```python
from build123d import *

# Parameters (mm, degrees)
BOSS_EXTRUDE2_DEPTH   = 3.81
BOSS_EXTRUDE2_2_DEPTH = 3.81
BOSS_EXTRUDE3_START   = 0.508
SKETCH2_3_R           = 2.794
BOSS_EXTRUDE3_DEPTH   = 2.286
BOSS_EXTRUDE11_DEPTH  = 3.81
BOSS_EXTRUDE12_DEPTH  = 0.889
BOSS_EXTRUDE14_START  = 10.16
BOSS_EXTRUDE14_DEPTH  = 50.8
BOSS_EXTRUDE17_START  = 60.071
BOSS_EXTRUDE17_DEPTH  = 0.889
SKETCH14_W            = 15.24
SKETCH14_H            = 59.182
CUT_EXTRUDE3_DEPTH    = 88.666803866


with BuildPart() as part:
    # Sketch2 → Boss-Extrude2 (new body)
    with BuildSketch(Plane(origin=(0, 0, 0), x_dir=(1, 0, 0), z_dir=(0, 1, 0))):
        Polygon((0, 7.62), (0, 0), (36.83, 0), (36.83, 7.62), (7.62, 7.62), (6.87, 7.62), align=None)
    extrude(amount=BOSS_EXTRUDE2_DEPTH)



with BuildPart() as body_2:
    # Sketch2 → Boss-Extrude2 2 (new body)
    with BuildSketch(Plane(origin=(0, 0, 0), x_dir=(1, 0, 0), z_dir=(0, 1, 0))):
        Polygon((0, 76.2), (0, 68.58), (6.87, 68.58), (7.62, 68.58), (36.83, 68.58), (36.83, 76.2), align=None)
    extrude(amount=BOSS_EXTRUDE2_2_DEPTH)


with BuildPart() as part_1:
    add(part.part)

    add(body_2.part)  # Boss-Extrude3 merges body 2
    # Sketch2<3> → Boss-Extrude3 (add)
    # profile 1 of 2: a face of its own
    with BuildSketch(Plane(origin=(0, 0, 0), x_dir=(1, 0, 0), z_dir=(0, 1, 0)).offset(BOSS_EXTRUDE3_START)):
        Polygon((0, 68.58), (0, 7.62), (6.87, 7.62), (7.62, 7.62), (36.83, 7.62), (36.83, 68.58), (7.62, 68.58), (6.87, 68.58), align=None)
        with Locations(Location((29.21, 22.86, 0), (0, 0, 270))):
            Circle(SKETCH2_3_R, mode=Mode.SUBTRACT)
        with Locations(Location((29.21, 53.34, 0), (0, 0, 270))):
            Circle(SKETCH2_3_R, mode=Mode.SUBTRACT)
    # profile 2 of 2: a face of its own
    with BuildSketch(Plane(origin=(0, 0, 0), x_dir=(1, 0, 0), z_dir=(0, 1, 0)).offset(BOSS_EXTRUDE3_START)):
        Polygon((0, 68.58), (0, 7.62), (6.87, 7.62), (7.62, 7.62), (36.83, 7.62), (36.83, 68.58), (7.62, 68.58), (6.87, 68.58), align=None)
        with Locations(Location((29.21, 22.86, 0), (0, 0, 270))):
            Circle(SKETCH2_3_R, mode=Mode.SUBTRACT)
        with Locations(Location((29.21, 53.34, 0), (0, 0, 270))):
            Circle(SKETCH2_3_R, mode=Mode.SUBTRACT)
    extrude(amount=BOSS_EXTRUDE3_DEPTH)

    # Sketch13 → Boss-Extrude11 (add)
    with BuildSketch(Plane.XY.offset(-68.58)):
        Polygon((6.215980089, 2.794), (7.231980089, 2.794), (7.231980089, 3.298518966), align=None)
        Polygon((8.120980089, 2.794), (8.120980089, 3.81), (7.231980089, 3.81), (7.231980089, 3.298518966), (7.231980089, 2.794), align=None)
        Polygon((8.120980089, 3.81), (8.120980089, 22.975432281), (8.120980089, 24.638), (9.046534916, 24.638), (19.649280137, 24.638), (20.820980089, 24.638), (21.060045846, 22.582034491), (23.242840554, 3.81), (24.261745737, 3.81), (21.784207173, 25.654), (7.231980089, 25.654), (7.231980089, 3.81), align=None)
        Polygon((8.120980089, 24.638), (8.120980089, 22.975432281), (9.046534916, 24.638), align=None)
        Polygon((20.820980089, 24.638), (19.649280137, 24.638), (21.060045846, 22.582034491), align=None)
        Polygon((24.261745737, 3.81), (23.242840554, 3.81), (23.360980089, 2.794), (24.376980089, 2.794), (24.307041878, 3.410632288), align=None)
        Polygon((24.307041878, 3.410632288), (24.376980089, 2.794), (25.392980089, 2.794), align=None)
    extrude(amount=BOSS_EXTRUDE11_DEPTH)

    # Sketch13<3> → Boss-Extrude12 (add)
    with BuildSketch(Plane.XY.offset(-68.58)):
        Polygon((9.046534916, 24.638), (8.120980089, 22.975432281), (8.120980089, 3.81), (23.242840554, 3.81), (21.060045846, 22.582034491), (19.649280137, 24.638), align=None)
        Polygon((23.242840554, 3.81), (8.120980089, 3.81), (8.120980089, 2.794), (23.360980089, 2.794), align=None)
    extrude(amount=BOSS_EXTRUDE12_DEPTH)

    # Sketch13<6> → Boss-Extrude14 (add)
    with BuildSketch(Plane.XY.offset(-68.58).offset(BOSS_EXTRUDE14_START)):
        Polygon((24.307041878, 3.410632288), (24.376980089, 2.794), (25.392980089, 2.794), align=None)
        Polygon((24.261745737, 3.81), (23.242840554, 3.81), (23.360980089, 2.794), (24.376980089, 2.794), (24.307041878, 3.410632288), align=None)
        Polygon((8.120980089, 2.794), (8.120980089, 3.81), (7.231980089, 3.81), (7.231980089, 3.298518966), (7.231980089, 2.794), align=None)
        Polygon((6.215980089, 2.794), (7.231980089, 2.794), (7.231980089, 3.298518966), align=None)
        Polygon((8.120980089, 3.81), (8.120980089, 22.975432281), (8.120980089, 24.638), (9.046534916, 24.638), (19.649280137, 24.638), (20.820980089, 24.638), (21.060045846, 22.582034491), (23.242840554, 3.81), (24.261745737, 3.81), (21.784207173, 25.654), (7.231980089, 25.654), (7.231980089, 3.81), align=None)
        Polygon((20.820980089, 24.638), (19.649280137, 24.638), (21.060045846, 22.582034491), align=None)
        Polygon((8.120980089, 24.638), (8.120980089, 22.975432281), (9.046534916, 24.638), align=None)
    extrude(amount=BOSS_EXTRUDE14_DEPTH)

    # Sketch13<7> → Boss-Extrude17 (add)
    with BuildSketch(Plane.XY.offset(-68.58).offset(BOSS_EXTRUDE17_START)):
        Polygon((9.046534916, 24.638), (8.120980089, 22.975432281), (8.120980089, 3.81), (23.242840554, 3.81), (21.060045846, 22.582034491), (19.649280137, 24.638), align=None)
        Polygon((23.242840554, 3.81), (8.120980089, 3.81), (8.120980089, 2.794), (23.360980089, 2.794), align=None)
    extrude(amount=BOSS_EXTRUDE17_DEPTH)

    # Sketch14 → Cut-Extrude3 (cut, through all)
    with BuildSketch(Plane(origin=(0, 2.794, 0), x_dir=(1, 0, 0), z_dir=(0, 1, 0))):
        with Locations((15.740980089, 38.1)):
            Rectangle(SKETCH14_W, SKETCH14_H)
    extrude(amount=-CUT_EXTRUDE3_DEPTH, mode=Mode.SUBTRACT)


solid = part_1.part
```
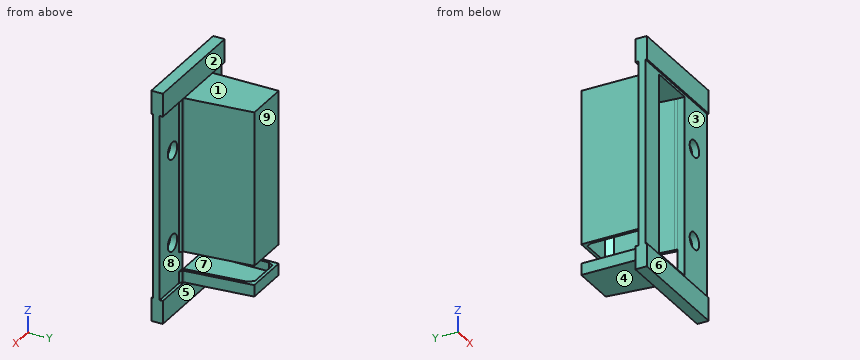
The listing builds one solid part. Answer for the finished solid, in the listing's coordinates (mm). Face numbers are marked on the shaded views. A direction names the side the tool comes from. Round coordinates to 2 decimals unless told otherwise and drop trailing zeros. Loops run counter-clockwise (first coordinate to the right, second up) from the corner with the lowest first, then second, coordinate; pieces in that order, holes last. Notation, with made-up numbers: (-8, 37) - (-3, 37) arc R9 ccw to (-3, 48) - close; hole circle Ø7 at (43, 74.25). An arc over 180 degrees is marked (long way). Return JSON: item names as keys, results as strings. Group by question number.
1. Each of these flat-tipped pins is pushed along its axis until it touches: P1, Ø6.5, axis at y = 12.5, z = -35.5, coming from the +X side; P2, Ø6, axis at x = 18, y = 19.5, coming from the +Z side; P3, Ø3, axis at x = 13.5, z = -66, coming from the -Y side. Where does it stop, or does it pass through?
2. The part is cut by section C-C on y = 13.25. Determine the outline of the cut face in (x, z).
3. The part is cut by section B-B on x = 12.5. Determine the outline of the cut face in (y, z).
4. The mould has two halves that part along Z. Classify the marked faces 1, 2, 3 and 4: pulls with the +Z half, pulls with the -Z half, needs draft (parallel to the pull), parting line crosses it, or undercut.
5. The part is cut by section D-D on x = 29.21. Determine the outline of the cut face in (y, z).
6. Which of the six approach directions +Z, -Z, +X, -X, +Y, -Y give full straight-line access (tool end or side, diameter ignored) to the marked faces 5, 6, 7, 8 and 9?
7. Consider probe 1 along X at (y, z) = (1, -22.86); probe 2 along Z at (x, y) = (14, 18); probe 3 along Z at (x, y) = (11.5, 1). Determine where each line is inside the solid, lowest interval first.
8. The part is cut by section A-A on z = -53.34. Determine the outline of the cut face in (x, y), then the cut area to 3 significant figures.
Resolved:
{
 "1": {"P1": "stops at x = 23.64", "P2": "stops at z = -7.62", "P3": "stops at y = 24.64"},
 "2": {"outline": "(7.23, -68.58) - (23.19, -68.58) - (23.19, -64.77) - (22.15, -64.77) - (22.15, -67.69) - (8.12, -67.69) - (8.12, -64.77) - (7.23, -64.77) - close; (7.23, -58.42) - (8.12, -58.42) - (8.12, -8.51) - (22.15, -8.51) - (22.15, -58.42) - (23.19, -58.42) - (23.19, -7.62) - (7.23, -7.62) - close"},
 "3": {"outline": "(0, -76.2) - (3.81, -76.2) - (3.81, -68.58) - (25.65, -68.58) - (25.65, -64.77) - (24.64, -64.77) - (24.64, -67.69) - (0.51, -67.69) - (0.51, -68.58) - (0, -68.58) - close; (0, -7.62) - (0.51, -7.62) - (0.51, -8.51) - (24.64, -8.51) - (24.64, -58.42) - (25.65, -58.42) - (25.65, -7.62) - (3.81, -7.62) - (3.81, 0) - (0, 0) - close"},
 "4": {"face 1": "pulls with the +Z half", "face 2": "needs draft", "face 3": "undercut", "face 4": "pulls with the -Z half"},
 "5": {"outline": "(0, -76.2) - (3.81, -76.2) - (3.81, -68.58) - (2.79, -68.58) - (2.79, -56.13) - (0.51, -56.13) - (0.51, -68.58) - (0, -68.58) - close; (0, -7.62) - (0.51, -7.62) - (0.51, -20.07) - (2.79, -20.07) - (2.79, -7.62) - (3.81, -7.62) - (3.81, 0) - (0, 0) - close; (0.51, -50.55) - (2.79, -50.55) - (2.79, -25.65) - (0.51, -25.65) - close"},
 "6": {"face 5": "-Z, +X, -X, +Y", "face 6": "+Z, -Z, +X, -X, -Y", "face 7": "-Y", "face 8": "+X, +Y", "face 9": "+Z, -Z, +X, -X, +Y"},
 "7": {"probe 1": "x = 0 to 8.12, 23.36 to 26.42, 32 to 36.83", "probe 2": "z = -68.58 to -67.69, -8.51 to -7.62", "probe 3": "z = -76.2 to -67.69, -8.51 to 0"},
 "8": {"outline": "(0, 0.51) - (8.12, 0.51) - (8.12, 22.98) - (9.05, 24.64) - (19.65, 24.64) - (21.06, 22.58) - (23.36, 2.79) - (23.36, 0.51) - (26.42, 0.51) - (26.42, 2.79) - (25.39, 2.79) - (24.31, 3.41) - (21.78, 25.65) - (7.23, 25.65) - (7.23, 3.3) - (6.22, 2.79) - (0, 2.79) - close; (32, 0.51) - (36.83, 0.51) - (36.83, 2.79) - (32, 2.79) - close", "area": "96.3 mm²"}
}
